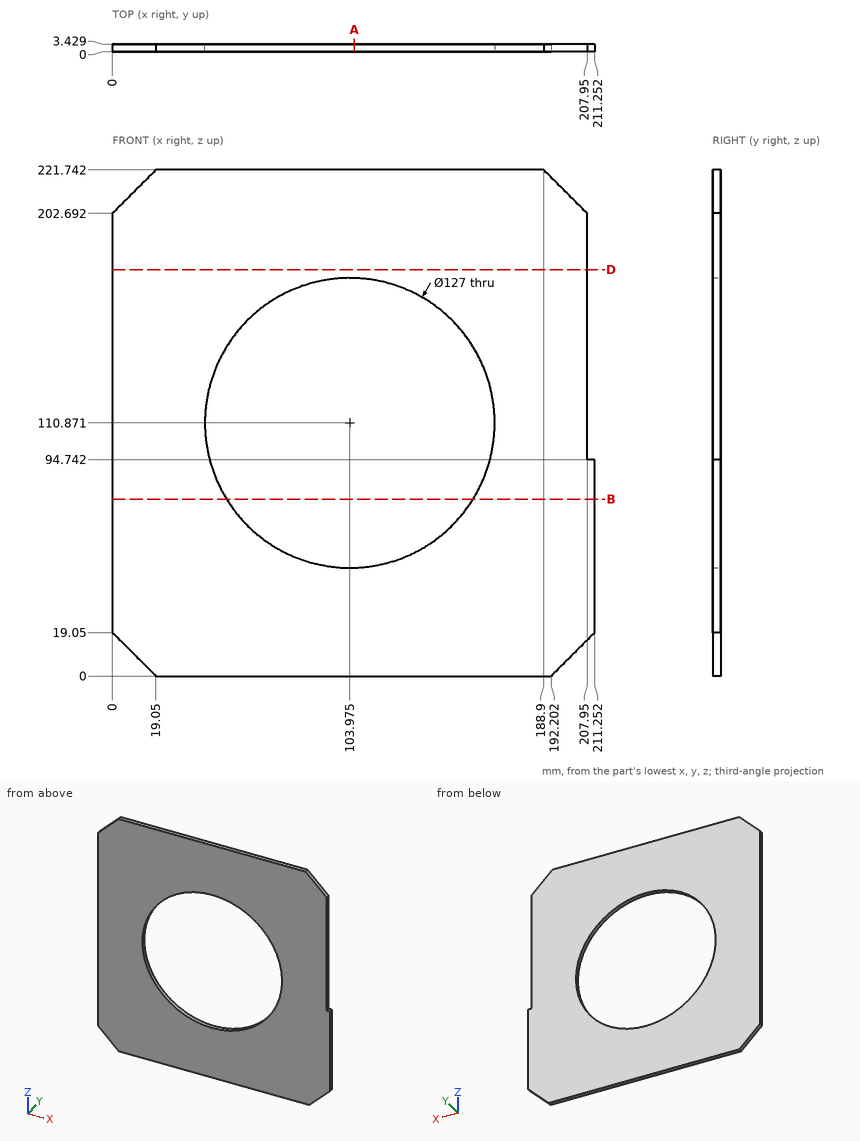
Here's the drawing with two shaded views (mm, measured from the low corner). I have some questions. Coordinates: 2 decimals unless noted, no trailing zeros. Order: outer loops, then holes, each group sorted by start corner. A loop starts at its lowest first (then second) coordinate and runs counter-clockwise, first axis right, second up. Notation, with made-up numbers: (53.25, -8) -> (104.25, -8) arc R17 cw to (104.25, 22) -> close; hole circle Ø2 at (85, 18). An arc over 180 degrees is marked (long way). Write each question's results on one line, items separated by ' | '.
Item 1: If I drill on line 1 along X through (y, z) = (2.4, 198.5); line 2 along Z through (x, y) = (81, 0.45); line 3 along X through (y, z) = (0.75, 75.5), over which ranges is the centre line in solid material (lowest first)?
Results are:
line 1: 0 to 207.95 | line 2: 0 to 51.67, 170.07 to 221.74 | line 3: 0 to 51.24, 156.71 to 211.25
Item 2: I'm going to push flat-ended pins straight in: pin 1 Ø1 at (x, y) = (210, 1.5) entering from +Z; pin 2 Ø1 at (y, z) = (1.5, 140.5) entering from +X. Where does each tip first touch, or does it pass through?
Results are:
pin 1: z = 94.74 | pin 2: x = 207.95
Item 3: I want a section at B-B, the plane z = 77.5. Write out the boundary of the cut face in (x, y).
Results are:
outline: (0, 0) -> (49.95, 0) -> (49.95, 3.43) -> (0, 3.43) -> close; (158, 0) -> (211.25, 0) -> (211.25, 3.43) -> (158, 3.43) -> close
Item 4: I want a section at D-D, the plane z = 178. Write out the boundary of the cut face in (x, y).
Results are:
outline: (0, 0) -> (207.95, 0) -> (207.95, 3.43) -> (0, 3.43) -> close
Item 5: I want a section at A-A, the plane x = 106. Write out the boundary of the cut face in (y, z), then the cut area to 3 significant figures.
Results are:
outline: (0, 0) -> (3.43, 0) -> (3.43, 47.4) -> (0, 47.4) -> close; (0, 174.34) -> (3.43, 174.34) -> (3.43, 221.74) -> (0, 221.74) -> close | area: 325 mm²
